```python
from build123d import *

# Parameters (mm, degrees)
F1_DEPTH = 12
F2_W     = 10
F2_H     = 10
F3_DEPTH = 0.5


with BuildPart() as f1:
    # F0 (on Right) → F1 (new body)
    with BuildSketch(Plane.YZ):
        Polygon((2.25, 16), (-2.25, 16), (-2.25, 14), (-0.25, 14), (-0.25, 2), (-2.25, 2), (-2.25, 0), (2.25, 0), (2.25, 2), (0.25, 2), (0.25, 14), (2.25, 14), align=None)
    extrude(amount=F1_DEPTH)

    # F2 (on face) → F3 (cut, through all)
    with BuildSketch(Plane(origin=(0, 0.25, 0), x_dir=(-1, 0, 0), z_dir=(0, 1, 0))):
        with Locations((-6, 8)):
            Rectangle(F2_W, F2_H)
    extrude(amount=-F3_DEPTH, mode=Mode.SUBTRACT)


solid = f1.part
```
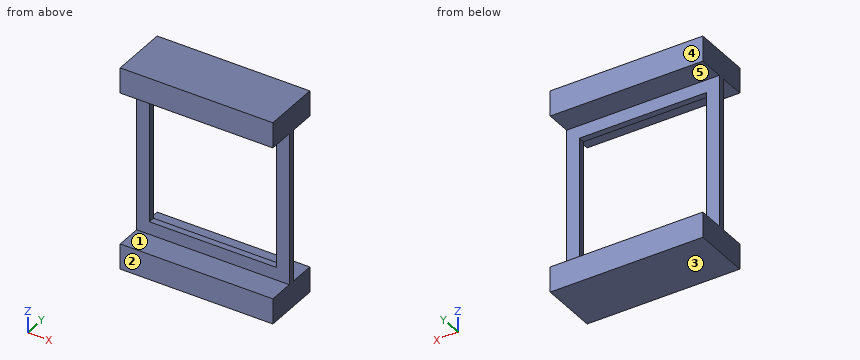
Read the model definition and answer for the solid it produces. Units are mm, in the model's axes. Face numbers are marked on the shaded views. A direction names the side the tool comes from. Give positions to 0.01 mm unless a question says otherwise; leave off trailing zeros. Order: outer loops, then holes, each group sorted by start corner. A loop starts at its lowest first (then second) coordinate and runs counter-clockwise, first axis right, second up. Notation, with made-up numbers: (66.25, 57) -> (114.25, 57) arc R26 ccw to (114.25, 72) -> close; hole circle Ø9 at (50, -40). An arc over 180 degrees is marked (long way). One line per item, written item: value. Start each with the question number.
(1) The part is cut by section D-D (z = 13.25). Determine the outline of the cut face in (x, y), and give its area (3 significant figures).
(2) The part is cut by section B-B (x = 1.5). Determine the outline of the cut face in (y, z), and give its area (3 significant figures).
(3) The part is cut by section A-A (y = 1.7). Determine the outline of the cut face in (x, z).
(4) Flat-ended cylindrical pins translate along their axes: P1, Ø6, axis at x = 3.5, z = 8, coming from the -Y side; P2, Ø1.5, axis at x = 5, z = 4, coming from the +Y side; P3, Ø5, axis at x = 2.5, z = 7, coming from the +Y side. Find the tip coordinate at first contact, or state that the pin passes through.
(5) The part is cut by section C-C (z = 11.5). Determine the outline of the cut face in (x, y).
(6) For a pull along Z with two mould halves and no side action, classify the marked faces 3, 4 and 5 as released by +Z, released by -Z, zero draft, split by the parting line, or undercut.
(7) Straight lines are drawn through the part: L1, parallel to Z at x = 3.75, y = 0; L2, parallel to Z at x = 3.5, y = -1.45; L3, parallel to X at y = 0.2, z = 6. For each, find the intervals that lie inside material, in ascending order.
(8) A tool of negligible diameter and unlimited length cuts with its end or side. For the marked faces 1 and 2, from which of +Z, -Z, +X, -X, +Y, -Y can it reach the whole face along a straight path? Write none if from no direction.
Taken from the geometry:
1. outline: (0, -0.25) -> (12, -0.25) -> (12, 0.25) -> (0, 0.25) -> close
1. area: 6.00 mm^2
2. outline: (-2.25, 0) -> (2.25, 0) -> (2.25, 2) -> (0.25, 2) -> (0.25, 3) -> (-0.25, 3) -> (-0.25, 2) -> (-2.25, 2) -> close; (-2.25, 14) -> (-0.25, 14) -> (-0.25, 13) -> (0.25, 13) -> (0.25, 14) -> (2.25, 14) -> (2.25, 16) -> (-2.25, 16) -> close
2. area: 19.0 mm^2
3. outline: (0, 0) -> (12, 0) -> (12, 2) -> (0, 2) -> close; (0, 14) -> (12, 14) -> (12, 16) -> (0, 16) -> close
4. P1: y = -0.25
4. P2: through
4. P3: y = 0.25
5. outline: (0, -0.25) -> (1, -0.25) -> (1, 0.25) -> (0, 0.25) -> close; (11, -0.25) -> (12, -0.25) -> (12, 0.25) -> (11, 0.25) -> close
6. face 3: released by -Z
6. face 4: zero draft
6. face 5: undercut
7. L1: 0 to 3, 13 to 16
7. L2: 0 to 2, 14 to 16
7. L3: 0 to 1, 11 to 12
8. face 1: +X, -X, -Y
8. face 2: +Z, -Z, +X, -X, -Y
